```python
from build123d import *

# Parameters (mm, degrees)
F0_R      = 10
F1_DEPTH  = 14
F2_R      = 6
F3_DEPTH  = 10
F4_R      = 5.5
F5_DEPTH  = 12.5
F6_DEPTH  = 9.25
F7_R      = 2
F8_DEPTH  = 12.5
F9_R      = 8
F10_DEPTH = 13
F11_R     = 5.5
F12_DEPTH = 0.5
F13_R     = 2
F14_DEPTH = 25


with BuildPart() as f1:
    # F0 (on Top) → F1 (new body)
    with BuildSketch(Plane.XY):
        Circle(F0_R)
    extrude(amount=F1_DEPTH)

    # F2 (on Front) → F3 (join, symmetric)
    with BuildSketch(Plane.XZ):
        with Locations((0, 7)):
            Circle(F2_R)
    extrude(amount=F3_DEPTH, both=True)

    # F4 (on Front) → F5 (cut, symmetric)
    with BuildSketch(Plane.XZ):
        with Locations((0, 7)):
            Circle(F4_R)
    extrude(amount=F5_DEPTH, both=True, mode=Mode.SUBTRACT)

    # F4 (on Front) → F6 (join, symmetric)
    with BuildSketch(Plane.XZ):
        with Locations((0, 7)):
            Circle(F4_R)
    extrude(amount=F6_DEPTH, both=True)

    # F7 (on Front) → F8 (cut, symmetric)
    with BuildSketch(Plane.XZ):
        with Locations((0, 7)):
            Circle(F7_R)
    extrude(amount=F8_DEPTH, both=True, mode=Mode.SUBTRACT)

    # F9 (on Top) → F10 (cut)
    with BuildSketch(Plane.XY):
        Circle(F9_R)
    extrude(amount=F10_DEPTH, mode=Mode.SUBTRACT)

    # F11 (on face) → F12 (cut)
    with BuildSketch(Plane.XY.offset(14)):
        Circle(F11_R)
    extrude(amount=-F12_DEPTH, mode=Mode.SUBTRACT)

    # F13 (on Top) → F14 (cut)
    with BuildSketch(Plane.XY):
        Circle(F13_R)
    extrude(amount=F14_DEPTH, mode=Mode.SUBTRACT)


solid = f1.part
```
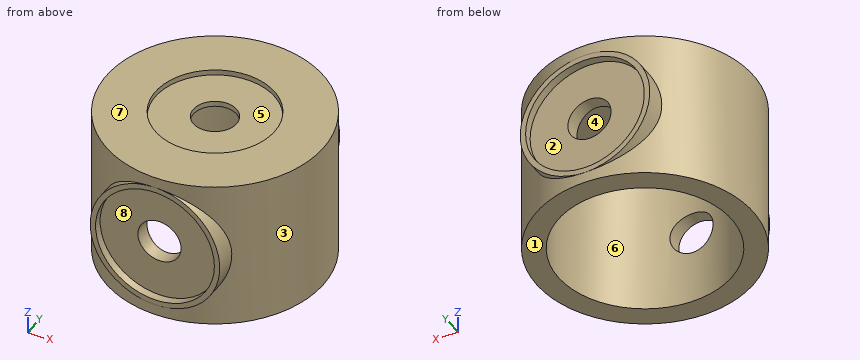
Work out the finished part from the listing and answer in its coordinate system (mm). Face numbers are marked on the shaded views. A direction names the side the tool comes from. Give positions to 0.01 mm unless a question says otherwise; leave off trailing zeros. Loops run counter-clockwise (first coordinate to the right, second up) from the corner with the lowest first, then second, coordinate; pieces in that order, holes last. Notation, with made-up numbers: (75.25, 67.25) -> (115.25, 67.25) arc R9 cw to (115.25, 76.25) -> close; hole circle Ø3 at (75, 87). An arc over 180 degrees is marked (long way). Write item = value, one per line. Start each with the question number.
(1) Find section D-D on x = -3.25. Give the vertices of the cut face in (y, z), and give its area (3 significant figures).
(2) Find section A-A on z = 7. Give the vertices of the cut face in (x, y).
(3) The mould has two halves that part along X. Classify the marked faces 1, 2, 3 and 4: +X half, -X half, draft (parallel to the pull), parting line (faces both ways), or undercut.
(4) Which of the six approach directions +Z, -Z, +X, -X, +Y, -Y give full straight-line access (tool end or side, diameter ignored) to the marked faces 5, 6, 7 and 8?
(5) Find section B-B on y = 0. Give the vertices of the cut face in (x, z), and give its area (3 significant figures).
(6) Find section C-C on z = 10.5. Give the vertices of the cut face in (x, y).
(7) Given pin 1 Ø4 at (y, z) = (5.5, 5) entering from +X; pin 2 Ø5.5 at (x, y) = (-2, 2) entering from +Z; pin 3 Ø5 at (x, z) = (0, 7) entering from -Y; pin 4 Ø2 at (y, z) = (1.5, 11.5) entering from -X, each flat-ended and moving along its own axis, determine where each tip first touches the part or whether it passes through.
(8) Find the intervals of material crossed by probe 1 along Z at (x, y) = (0, 9.55); probe 2 along Z at (x, y) = (0, 8.6); probe 3 along Y at (x, z) = (2, 5), in increasing order. Write a range as from..to.
From the geometry:
q1.outline = (-10, 1.96) -> (-9.46, 1.96) -> (-9.46, 0) -> (-7.31, 0) -> (-7.31, 13) -> (7.31, 13) -> (7.31, 0) -> (9.46, 0) -> (9.46, 1.96) -> (10, 1.96) -> (10, 2.56) -> (9.25, 2.56) -> (9.25, 11.44) -> (10, 11.44) -> (10, 12.04) -> (9.46, 12.04) -> (9.46, 14) -> (4.44, 14) -> (4.44, 13.5) -> (-4.44, 13.5) -> (-4.44, 14) -> (-9.46, 14) -> (-9.46, 12.04) -> (-10, 12.04) -> (-10, 11.44) -> (-9.25, 11.44) -> (-9.25, 2.56) -> (-10, 2.56) -> close
q1.area = 67.9 mm^2
q2.outline = (-6, -10) -> (-5.5, -10) -> (-5.5, -9.25) -> (-2, -9.25) -> (-2, -7.75) arc R8 cw to (-2, 7.75) -> (-2, 9.25) -> (-5.5, 9.25) -> (-5.5, 10) -> (-6, 10) -> (-6, 8) arc R10 ccw to (-6, -8) -> close; (2, -9.25) -> (5.5, -9.25) -> (5.5, -10) -> (6, -10) -> (6, -8) arc R10 ccw to (6, 8) -> (6, 10) -> (5.5, 10) -> (5.5, 9.25) -> (2, 9.25) -> (2, 7.75) arc R8 cw to (2, -7.75) -> close
q3.face_1 = draft
q3.face_2 = undercut
q3.face_3 = parting line
q3.face_4 = undercut
q4.face_5 = +Z
q4.face_6 = -Z
q4.face_7 = +Z, +X, -X, +Y, -Y
q4.face_8 = -Y
q5.outline = (-10, 0) -> (-8, 0) -> (-8, 13) -> (-2, 13) -> (-2, 13.5) -> (-5.5, 13.5) -> (-5.5, 14) -> (-10, 14) -> close; (2, 13) -> (8, 13) -> (8, 0) -> (10, 0) -> (10, 14) -> (5.5, 14) -> (5.5, 13.5) -> (2, 13.5) -> close
q5.area = 64.5 mm^2
q6.outline = (-4.87, -10) -> (-4.24, -10) -> (-4.24, -9.25) -> (4.24, -9.25) -> (4.24, -10) -> (4.87, -10) -> (4.87, -8.73) arc R10 ccw to (4.87, 8.73) -> (4.87, 10) -> (4.24, 10) -> (4.24, 9.25) -> (-4.24, 9.25) -> (-4.24, 10) -> (-4.87, 10) -> (-4.87, 8.73) arc R10 ccw to (-4.87, -8.73) -> close; hole circle Ø16 at (0, 0)
q7.pin_1 = 9.37
q7.pin_2 = 14
q7.pin_3 = -9.25
q7.pin_4 = -9.99
q8.probe_1 = 0..1.5, 12.5..14
q8.probe_2 = 0..5, 9..14
q8.probe_3 = -9.25..-7.75, 7.75..9.25
